from build123d import *

# Parameters (mm, degrees)
SKETCH1_W           = 254
SKETCH1_H           = 69.85
BOSS_EXTRUDE1_DEPTH = 2.3622
SKETCH2_W           = 38.1
SKETCH2_H           = 25.4
CUT_EXTRUDE1_DEPTH  = 264.439940952
SKETCH3_R           = 3.2639
CUT_EXTRUDE2_DEPTH  = 264.439940952


with BuildPart() as part:
    # Sketch1 → Boss-Extrude1 (new body)
    with BuildSketch(Plane.XY):
        with Locations((127, 34.925)):
            Rectangle(SKETCH1_W, SKETCH1_H)
    extrude(amount=BOSS_EXTRUDE1_DEPTH)

    # Sketch2 → Cut-Extrude1 (cut, through all)
    with BuildSketch(Plane.XY.offset(2.3622)):
        with Locations((19.05, 34.925)):
            Rectangle(SKETCH2_W, SKETCH2_H)
    extrude(amount=-CUT_EXTRUDE1_DEPTH, mode=Mode.SUBTRACT)

    # Sketch3 → Cut-Extrude2 (cut, through all)
    with BuildSketch(Plane.XY.offset(2.3622)):
        with Locations((12.7, 62.23)):
            Circle(SKETCH3_R)
    extrude(amount=-CUT_EXTRUDE2_DEPTH, mode=Mode.SUBTRACT)


solid = part.part
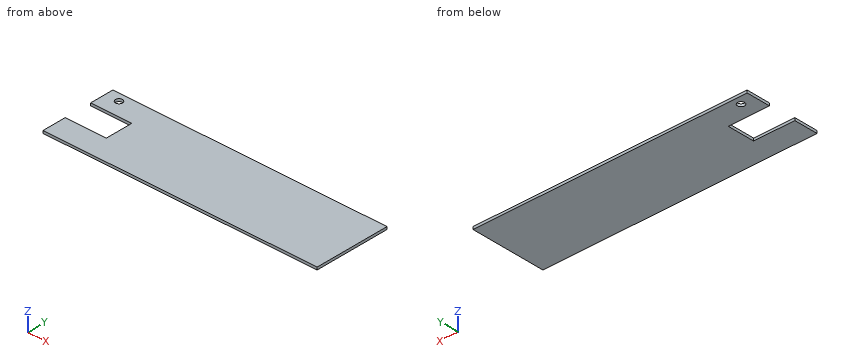
Work out the finished part from the listing and answer in its coordinate system (mm). Give positions to 0.01 mm unless a question says otherwise; leave off trailing zeros. Loops run counter-clockwise (first coordinate to the right, second up) from the corner with the lowest first, then second, coordinate; pieces in that order, holes last. Notation, with made-up numbers: (19, 1.5) -> (39, 1.5) arc R17 ccw to (39, 27.5) -> close; hole circle Ø9 at (54, 85.5). An arc over 180 degrees is marked (long way). Use a Markdown table: item, result. Add a question column.
1. Find the intervals of material crossed by probe 1 along Y at (x, z) = (12.7, 1.25) (3 decimals); probe 2 along X at (y, z) = (31, 2), in increasing order.
2. Section C-C on z = 2 is taken. Determine the outline of the cut face in (x, y) (3 decimals).
3. A flat-ended cylindrical pin translates along its axis: pin 1 Ø1.2 at (y, z) = (34, 1) entering from -X. Find the tip coordinate at first contact, or state that the pin passes through.
4. Section B-B on y = 62.23 is taken. Determine the outline of the cut face in (x, z), and give its area (3 significant figures).
5. Section A-A on x = 12.7 is taken. Determine the outline of the cut face in (y, z) (3 decimals), and give its area (3 significant figures).
6. Section D-D on y = 32 is taken. Determine the outline of the cut face in (x, z), and give its area (3 significant figures).
Results below:
| question | item | result |
|---|---|---|
| 1 | probe 1 | y = 0 to 22.225, 47.625 to 58.966, 65.494 to 69.85 |
| 1 | probe 2 | x = 38.1 to 254 |
| 2 | outline | (0, 0) -> (254, 0) -> (254, 69.85) -> (0, 69.85) -> (0, 47.625) -> (38.1, 47.625) -> (38.1, 22.225) -> (0, 22.225) -> close; hole circle Ø6.528 at (12.7, 62.23) |
| 3 | pin 1 | stops at x = 38.1 |
| 4 | outline | (0, 0) -> (9.44, 0) -> (9.44, 2.36) -> (0, 2.36) -> close; (15.96, 0) -> (254, 0) -> (254, 2.36) -> (15.96, 2.36) -> close |
| 4 | area | 585 mm^2 |
| 5 | outline | (0, 0) -> (22.225, 0) -> (22.225, 2.362) -> (0, 2.362) -> close; (47.625, 0) -> (58.966, 0) -> (58.966, 2.362) -> (47.625, 2.362) -> close; (65.494, 0) -> (69.85, 0) -> (69.85, 2.362) -> (65.494, 2.362) -> close |
| 5 | area | 89.6 mm^2 |
| 6 | outline | (38.1, 0) -> (254, 0) -> (254, 2.36) -> (38.1, 2.36) -> close |
| 6 | area | 510 mm^2 |
